```python
from build123d import *

# Parameters (mm, degrees)
SKETCH1_W                = 195.277
SKETCH1_H                = 70
MAIN_DEPTH               = 1.1811
ANGLECUTS_REACH          = 105.749
BRACKETHOLES_D           = 3.5
BRACKETHOLES_DEPTH       = 5
BRACKETHOLES_CSINK_D     = 6.3
BRACKETHOLES_CSINK_ANGLE = 90


with BuildPart() as part:
    # Sketch1 → Main (new, symmetric)
    with BuildSketch(Plane.XY):
        Rectangle(SKETCH1_W, SKETCH1_H)
    extrude(amount=MAIN_DEPTH, both=True)

    # Sketch2 → AngleCuts (cut, up to next)
    with BuildSketch(Plane.XY.offset(1.1811), mode=Mode.PRIVATE) as anglecuts_sk1:
        Polygon((-97.6385, 35), (-72.160583601, 35), (-97.6385, -35), align=None)
    anglecuts_tool1 = extrude(anglecuts_sk1.sketch, amount=-ANGLECUTS_REACH, mode=Mode.PRIVATE) & part.part
    # Sketch2 → AngleCuts (cut, up to next)
    with BuildSketch(Plane.XY.offset(1.1811), mode=Mode.PRIVATE) as anglecuts_sk2:
        Polygon((97.6385, 35), (97.6385, -35), (72.160583601, 35), align=None)
    anglecuts_tool2 = extrude(anglecuts_sk2.sketch, amount=-ANGLECUTS_REACH, mode=Mode.PRIVATE) & part.part
    add(anglecuts_tool1.solids().sort_by_distance((-89.145861, 11.666667, 1.1811))[0], mode=Mode.SUBTRACT)
    add(anglecuts_tool2.solids().sort_by_distance((89.145861, 11.666667, 1.1811))[0], mode=Mode.SUBTRACT)

    # BracketHoles
    with Locations(Plane.XY.offset(1.1811)):
        with Locations((-72.6378, -15), (-57.6378, 11.3815573), (57.6378, 11.3815573), (72.6378, -15)):
            CounterSinkHole(BRACKETHOLES_D / 2, BRACKETHOLES_CSINK_D / 2, depth=BRACKETHOLES_DEPTH, counter_sink_angle=BRACKETHOLES_CSINK_ANGLE)


solid = part.part
```
For this review, take the finished solid that the model builds, in its own axes (mm). Give positions to 0.01 mm unless a question says otherwise; leave off trailing zeros. Write each loop counter-clockwise with the first axis right and the second up, starting at its lowest first coordinate (ties: lowest second). Pieces come first, ordered by that corner, then holes. Notation, with made-up numbers: M -22.5,-5 L 13.5,-5 A23 cw 13.5,14 Z; hole C 56,87.5 d1. An arc over 180 degrees is marked long. Answer as CSV lines item,"result".
1. Draft analysis for pull direction Y (two halves, no side actions). For faces 1 (the cylindrical face through (56.02, 10.71, -0.71)), 2 (the flat face through (-1, 0, -1.181)), 3 (the flat face through (-84.72, 0.49, 0.02)), state which applies: +Y half, -Y half, draft (parallel to the pull), parting line (faces both ways), or undercut.
Findings:
face 1,"undercut"
face 2,"draft"
face 3,"+Y half"
2. Consider section C-C, the plane y = -29.5. Write out the cut boundary in (x, z), then the cut area to 3 significant figures.
Findings:
outline,"M -95.64,-1.18 L 95.64,-1.18 L 95.64,1.18 L -95.64,1.18 Z"
area,"452 mm2"
3. Consider section D-D, the plane y = -4. Write out the cut boundary in (x, z).
Findings:
outline,"M -86.36,-1.18 L 86.36,-1.18 L 86.36,1.18 L -86.36,1.18 Z"
4. For pin 1 (1 mm diameter, centred on y = -10, z = 0, fed in from +X), flat-tipped, find the tip position at first contact; note if it passes through.
Findings:
pin 1,"stops at x = 88.72"
5. Wall thickness on line 1 (Y direction, x = 57.5, z = -0.55); line 2 (X direction, y = -15, z = -0.4); line 3 (X direction, y = -26.5, z = 0.9): over which ranges is each line inside the solid? List them lowest first.
Findings:
line 1,"y = -35 to 9.64, 13.13 to 35"
line 2,"x = -90.36 to -74.39, -70.89 to 70.89, 74.39 to 90.36"
line 3,"x = -94.54 to 94.54"
6. Consider section B-B, the plane y = -15. Write out the cut boundary in (x, z).
Findings:
outline,"M -90.36,-1.18 L -74.39,-1.18 L -74.39,-0.22 L -75.79,1.18 L -90.36,1.18 Z; M -70.89,-1.18 L 70.89,-1.18 L 70.89,-0.22 L 69.49,1.18 L -69.49,1.18 L -70.89,-0.22 Z; M 74.39,-1.18 L 90.36,-1.18 L 90.36,1.18 L 75.79,1.18 L 74.39,-0.22 Z"
7. Consider section A-A, the plane z = -0.6. Write out the cut boundary in (x, y).
Findings:
outline,"M -97.64,-35 L 97.64,-35 L 72.16,35 L -72.16,35 Z; hole C -72.64,-15 d3.5; hole C -57.64,11.38 d3.5; hole C 57.64,11.38 d3.5; hole C 72.64,-15 d3.5"
